Geometry: see drawing. Coordinates: mm, zero at the bounding-box minimum. A direction names the side the tool comes from. Give positions to 0.01 mm unless a question says otherwise; leave off trailing zeros. Write each loop counter-clockwise with the first axis right and the second up, starting at its lowest first coordinate (ties: lowest second). Pieces come first, ordered by that corner, then holes. Notation, with made-up numbers: M 30.25,23 L 49.25,23 A7 cw 49.25,28 Z; hole C 31.25,-38.5 d10. An arc over 180 degrees is marked long. Use a Markdown table: item, result. Add a question column.
1) Line query: line 1 (Y direction, x = 5.5, z = 1.1) (1 decimal); line 2 (Y direction, x = 4, z = 1.55) (1 decimal); line 3 (X direction, y = 2.5, z = 3.8) (1 decimal). Output: solid intervals per line, ascending.
2) Section D-D on x = 1.5. Return the cut outline in (y, z) (1 decimal), then the cut area to 3 significant figures.
3) Set-up query: the marked faces 4 and 5. Return all of +Z, -Z, +X, -X, +Y, -Y with unobstructed straight access to the full face (end or side cutting, diameter ignored); none if empty.
4) Pin query (flat end, axial travel): pin 1 (1 mm diameter, centred on y = 4, z = 2, fed in from -X). Return the tip coordinate at first contact, or that it passes through.
5) Section C-C on z = 3.4. Return the cut outline in (x, y).
6) Draft query along X for the marked faces 1, 2 and 3. Return one class per face: +X half, -X half, draft (parallel to the pull), parting line (faces both ways), or undercut.
7) Section B-B on x = 8. Return the cut outline in (y, z) (1 decimal), then the cut area to 3 significant figures.
8) Section A-A on y = 2.25. Return the cut outline in (x, z) (1 decimal), then the cut area to 3 significant figures.
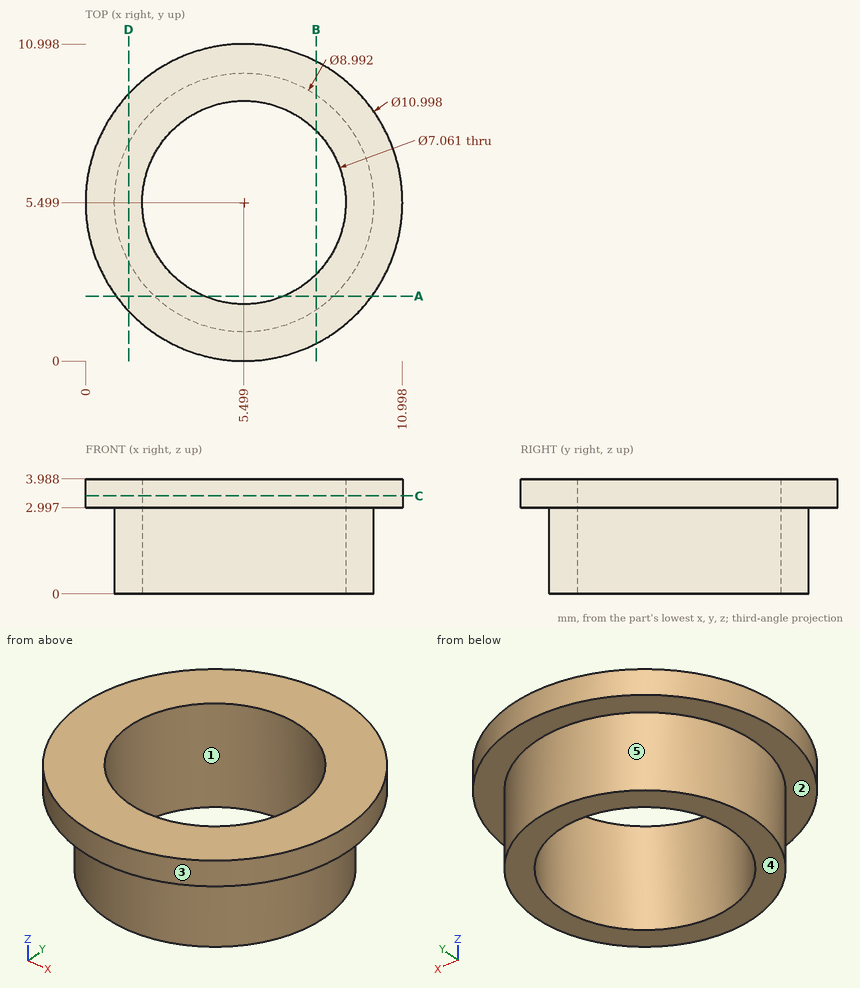
Found:
| question | item | result |
|---|---|---|
| 1 | line 1 | 1 to 2, 9 to 10 |
| 1 | line 2 | 1.3 to 2.3, 8.7 to 9.7 |
| 1 | line 3 | 0.9 to 3.6, 7.4 to 10.1 |
| 2 | outline | M 1.7,3 L 3.4,3 L 3.4,0 L 7.6,0 L 7.6,3 L 9.3,3 L 9.3,4 L 1.7,4 Z |
| 2 | area | 19.8 mm² |
| 3 | face 4 | -Z, +X, -X, +Y, -Y |
| 3 | face 5 | -Z |
| 4 | pin 1 | x = 1.12 |
| 5 | outline | C 5.5,5.5 d11; hole C 5.5,5.5 d7.06 |
| 6 | face 1 | undercut |
| 6 | face 2 | draft |
| 6 | face 3 | parting line |
| 7 | outline | M 0.6,3 L 1.8,3 L 1.8,0 L 3,0 L 3,4 L 0.6,4 Z; M 8,0 L 9.2,0 L 9.2,3 L 10.4,3 L 10.4,4 L 8,4 Z |
| 7 | area | 12.2 mm² |
| 8 | outline | M 1.1,3 L 2.4,3 L 2.4,0 L 4.1,0 L 4.1,4 L 1.1,4 Z; M 6.9,0 L 8.6,0 L 8.6,3 L 9.9,3 L 9.9,4 L 6.9,4 Z |
| 8 | area | 16.4 mm² |
